The model under review builds one solid part; all positions refer to its coordinate system, in mm. A direction names the side the tool comes from. Round coordinates to 2 decimals unless told otherwise and drop trailing zeros. Order: outer loops, then holes, each group sorted by start corner. A loop starts at its lowest first (then second) coordinate and runs counter-clockwise, first axis right, second up. Notation, with made-up numbers: M -35,-1.75 L 2,-1.75 A10 ccw 2,6.25 Z; hole C 17,11.5 d11. An arc over 180 degrees is marked long. Answer as CSV lines item,"result". Start each with the question number.
from build123d import *

# Parameters (mm, degrees)
CROQUIS1_R              = 4
CROQUIS1_R_2            = 1.25
SALIENTE_EXTRUIR1_DEPTH = 2.5
REDONDEO1_R             = 2.5


with BuildPart() as part:
    # Croquis1 → Saliente-Extruir1 (new, symmetric)
    # profile 1 of 4: a face of its own
    with BuildSketch(Plane(origin=(0, 0, 0), x_dir=(1, 0, 0), z_dir=(0, 1, 0))):
        with BuildLine():
            Line((-13.68, 17.49), (-13.68, -11.932810861))
            ThreePointArc((-13.68, -11.932810861), (-11.43, -11.24), (-9.18, -11.932810861))
            Line((-9.18, -11.932810861), (-9.18, 12.99))
            Line((-9.18, 12.99), (8.122810861, 12.99))
            ThreePointArc((8.122810861, 12.99), (7.43, 15.24), (8.122810861, 17.49))
            Line((8.122810861, 17.49), (-13.68, 17.49))
        make_face()
    # profile 2 of 4: a face of its own
    with BuildSketch(Plane(origin=(0, 0, 0), x_dir=(1, 0, 0), z_dir=(0, 1, 0))):
        with BuildLine():
            ThreePointArc((-7.43, -15.24), (-7.607124344, -16.417124344), (-8.122810861, -17.49))
            Line((-8.122810861, -17.49), (13.68, -17.49))
            Line((13.68, -17.49), (13.68, 11.932810861))
            ThreePointArc((13.68, 11.932810861), (11.43, 11.24), (9.18, 11.932810861))
            Line((9.18, 11.932810861), (9.18, -12.99))
            Line((9.18, -12.99), (-8.122810861, -12.99))
            ThreePointArc((-8.122810861, -12.99), (-7.607124344, -14.062875656), (-7.43, -15.24))
        make_face()
    # profile 3 of 4: a face of its own
    with BuildSketch(Plane(origin=(0, 0, 0), x_dir=(1, 0, 0), z_dir=(0, 1, 0))):
        with Locations((11.43, 15.24)):
            Circle(CROQUIS1_R)
        with Locations(Location((11.43, 15.24, 0), (0, 0, 270))):
            Circle(CROQUIS1_R_2, mode=Mode.SUBTRACT)
    # profile 4 of 4: a face of its own
    with BuildSketch(Plane(origin=(0, 0, 0), x_dir=(1, 0, 0), z_dir=(0, 1, 0))):
        with Locations((-11.43, -15.24)):
            Circle(CROQUIS1_R)
        with Locations(Location((-11.43, -15.24, 0), (0, 0, 270))):
            Circle(CROQUIS1_R_2, mode=Mode.SUBTRACT)
    extrude(amount=SALIENTE_EXTRUIR1_DEPTH, both=True)

    # Redondeo1
    redondeo1_edges = [part.edges().sort_by_distance(p)[0] for p in [
        (-9.18, 0, -12.99),
        (9.18, 0, 12.99),
        (13.68, 0, 17.49),
        (-13.68, 0, -17.49),
    ]]
    fillet(redondeo1_edges, radius=REDONDEO1_R)


solid = part.part
Item 1: Wall thickness on probe 1 along Z at (x, y) = (4, -1.8); probe 2 along X at (y, z) = (-1.75, 8); probe 3 along X at (y, z) = (-1.45, 11): over which ranges is each line inside the solid? List them lowest first. Write a range as [from, to].
Item 2: Consider section D-D (z = -13.5). State the section outline as (x, y) points, and give its area (3 significant figures).
Item 3: Consider section A-A (x = 1). State the section outline as (y, z) points, and give its area (3 significant figures).
Item 4: Consider section B-B (y = -0.2). State the section outline as (x, z) points.
Item 5: Consider section C-C (z = -1.5). State the section outline as (x, y) points, and give its area (3 significant figures).
Item 6: For pin 1 (1 mm diameter, centred on y = -1, z = -14, fed in from +X); pin 2 (2.5 mm diameter, centred on x = 2, y = 0.5, fed in from +Z); pin 3 (2 mm diameter, centred on x = -11.43, z = 15.24, fed in from -Y); pin 4 (2.5 mm diameter, centred on x = -3.5, y = -0.5, fed in from -Z), all flat-tipped, find the tip position at first contact; note any pin that passes through.
Item 7: The part is to be moulded in two halves that separate along X. For faces 4 (the cylindrical face through (12.967, 0.035, 16.738)), 5 (the flat face through (1, 0, 17.49)), 6 (the cylindrical face through (-8.428, 0.035, -12.277)), say which applies: +X half, -X half, draft (parallel to the pull), parting line (faces both ways), or undercut.
Item 8: Tool access review of faces 1 (the cylindrical face through (8.594, 0.035, -12.419)), 2 (the flat face through (13.68, 0, 2)), 3 (the flat face through (-1, 0, -17.49)): name each direction out of +Z, -Z, +X, -X, +Y, -Y from which nothing blocks a thin tool from reaching the whole face with its end or side.
Reported:
1,probe 1,"z = [-17.49, -12.99], [12.99, 17.49]"
1,probe 2,"x = [-13.68, -9.18], [9.18, 13.68]"
1,probe 3,"x = [-13.68, -9.18], [9.13, 13.68]"
2,outline,"M -13.68,-2.5 L 15.03,-2.5 L 15.03,2.5 L -13.68,2.5 Z"
2,area,"144 mm²"
3,outline,"M -2.5,-17.49 L 2.5,-17.49 L 2.5,-12.99 L -2.5,-12.99 Z; M -2.5,12.99 L 2.5,12.99 L 2.5,17.49 L -2.5,17.49 Z"
3,area,"45.0 mm²"
4,outline,"M -13.68,-14.99 A2.5 ccw -11.18,-17.49 L 8.12,-17.49 A4 ccw long 13.68,-11.93 L 13.68,14.99 A2.5 ccw 11.18,17.49 L -8.12,17.49 A4 ccw long -13.68,11.93 Z; hole C -11.43,15.24 d2.5; hole M -9.18,-10.49 A2.5 ccw -6.68,-12.99 L 8.12,-12.99 A4 cw 9.18,-11.93 L 9.18,10.49 A2.5 ccw 6.68,12.99 L -8.12,12.99 A4 cw -9.18,11.93 Z; hole C 11.43,-15.24 d2.5"
5,outline,"M -13.68,-2.5 L -9.18,-2.5 L -9.18,2.5 L -13.68,2.5 Z; M 9.18,-2.5 L 13.68,-2.5 L 13.68,2.5 L 9.18,2.5 Z"
5,area,"45.0 mm²"
6,pin 1,"stops at x = 15.36"
6,pin 2,"stops at z = 17.49"
6,pin 3,"passes through"
6,pin 4,"stops at z = -17.49"
7,face 4,"+X half"
7,face 5,"draft"
7,face 6,"undercut"
8,face 1,"+Y, -Y"
8,face 2,"+Z, +X, +Y, -Y"
8,face 3,"-Z, -X, +Y, -Y"
